Verification items for the finished model (mm, model axes). A direction names the side the tool comes from. Round coordinates to 2 decimals unless told otherwise and drop trailing zeros. Loops run counter-clockwise (first coordinate to the right, second up) from the corner with the lowest first, then second, coordinate; pieces in that order, holes last. Notation, with made-up numbers: (38.25, 28.5) -> (52.25, 28.5) arc R27 ccw to (52.25, 59.5) -> close; hole circle Ø2 at (-10.5, 44). An arc over 180 degrees is marked (long way). Write item = value, one per line. Start each with the question number.
```python
from build123d import *

# Parameters (mm, degrees)
SKETCH1_W           = 63.5
SKETCH1_H           = 38.1
BOSS_EXTRUDE1_DEPTH = 19.05
SHELL1_T            = -2.54
SKETCH2_R           = 1.143
CUT_EXTRUDE1_DEPTH  = 54.127911685
SKETCH4_W           = 7.62
SKETCH4_H           = 12.842115784
CUT_EXTRUDE2_DEPTH  = 54.127911685
SKETCH5_R           = 2.667
CUT_EXTRUDE3_DEPTH  = 54.127911685
SKETCH6_W           = 27.94
SKETCH6_H           = 27.94
CUT_EXTRUDE4_DEPTH  = 69.978656119


with BuildPart() as part:
    # Sketch1 → Boss-Extrude1 (new, symmetric)
    with BuildSketch(Plane.XY):
        Rectangle(SKETCH1_W, SKETCH1_H)
    extrude(amount=BOSS_EXTRUDE1_DEPTH, both=True)

    # Shell1
    shell1_openings = [part.faces().sort_by_distance(p)[0] for p in [
        (0, -19.05, 0),
    ]]
    offset(amount=SHELL1_T, openings=shell1_openings, kind=Kind.INTERSECTION)

    # Sketch2 → Cut-Extrude1 (cut, through all)
    with BuildSketch(Plane(origin=(0, 19.05, 0), x_dir=(1, 0, 0), z_dir=(0, 1, 0))):
        with Locations(Location((-1.27, 10.414, 0), (0, 0, 270))):
            Circle(SKETCH2_R)
        with Locations(Location((21.59, 10.414, 0), (0, 0, 270))):
            Circle(SKETCH2_R)
        with Locations(Location((21.59, -10.414, 0), (0, 0, 270))):
            Circle(SKETCH2_R)
        with Locations(Location((-1.27, -10.414, 0), (0, 0, 270))):
            Circle(SKETCH2_R)
    extrude(amount=-CUT_EXTRUDE1_DEPTH, mode=Mode.SUBTRACT)

    # Sketch4 → Cut-Extrude2 (cut, through all)
    with BuildSketch(Plane(origin=(0, 19.05, 0), x_dir=(1, 0, 0), z_dir=(0, 1, 0))):
        with Locations((-21.59, 0)):
            Rectangle(SKETCH4_W, SKETCH4_H)
    extrude(amount=-CUT_EXTRUDE2_DEPTH, mode=Mode.SUBTRACT)

    # Sketch5 → Cut-Extrude3 (cut, through all)
    with BuildSketch(Plane.XY.offset(19.05)):
        with Locations((-12.7, 0)):
            Circle(SKETCH5_R)
    extrude(amount=-CUT_EXTRUDE3_DEPTH, mode=Mode.SUBTRACT)

    # Sketch6 → Cut-Extrude4 (cut, through all)
    with BuildSketch(Plane.ZY.offset(31.75)):
        Rectangle(SKETCH6_W, SKETCH6_H)
    extrude(amount=-CUT_EXTRUDE4_DEPTH, mode=Mode.SUBTRACT)


solid = part.part
```
(1) Section check B-B on z = 1.5. Enter the section's corners in (x, y), then the cut area to 3 significant figures.
(2) Depth check by flat-ended pin: pin 1 Ø1.4 at (x, z) = (21.59, 10.414) entering from +Y; pin 2 Ø8 at (x, z) = (16.5, 7) entering from -Y. Enter the tip coordinate at first touch or a pass-through.
(3) Access from +Z, -Z, +X, -X, +Y, -Y to the whole of each face (thin tool, end or side, straight path). Record for faces 4 (the flat face through (-17.78, 18, 0)), 5 (the flat face through (30, 0, -13.97)), 6 (the flat face through (0, -1, -16.51)).
(4) Section check C-C on y = 0. Enter the section's corners in (x, z), then the cut area to 3 significant figures.
(5) Section check A-A on x = -12.7. Enter the section's corners in (y, z), then the cut area to 3 significant figures.
(6) Section check D-D on y = 5. Enter the section's corners in (x, z), then the cut area to 3 significant figures.
(7) Scan lines: line 1 (X direction, y = -5, z = -16); line 2 (Z direction, x = -6, y = -7); line 3 (Z direction, x = 21, y = 17). Record each from-to range of solid material in increasing order. Write a range as [from, to].
(8) Draft check along X on faces 1 (the flat face through (-22, 18, -6.421)), 2 (the flat face through (31.75, -17, 0)), 3 (the flat face through (0, 19.05, 0)). Enter one of: +X half, -X half, draft (parallel to the pull), parting line (faces both ways), or undercut.
Computed values:
q1.outline = (-31.75, -19.05) -> (-29.21, -19.05) -> (-29.21, -13.97) -> (-31.75, -13.97) -> close; (-31.75, 13.97) -> (-29.21, 13.97) -> (-29.21, 16.51) -> (-25.4, 16.51) -> (-25.4, 19.05) -> (-31.75, 19.05) -> close; (-17.78, 16.51) -> (29.21, 16.51) -> (29.21, 13.97) -> (31.75, 13.97) -> (31.75, 19.05) -> (-17.78, 19.05) -> close; (29.21, -19.05) -> (31.75, -19.05) -> (31.75, -13.97) -> (29.21, -13.97) -> close
q1.area = 181 mm²
q2.pin_1 = through
q2.pin_2 = 16.51
q3.face_4 = +Y, -Y
q3.face_5 = +X, -X
q3.face_6 = -Y
q4.outline = (-31.75, -19.05) -> (-15.37, -19.05) -> (-15.37, -16.51) -> (-29.21, -16.51) -> (-29.21, -13.97) -> (-31.75, -13.97) -> close; (-31.75, 13.97) -> (-29.21, 13.97) -> (-29.21, 16.51) -> (-15.37, 16.51) -> (-15.37, 19.05) -> (-31.75, 19.05) -> close; (-10.03, -19.05) -> (31.75, -19.05) -> (31.75, -13.97) -> (29.21, -13.97) -> (29.21, -16.51) -> (-10.03, -16.51) -> close; (-10.03, 16.51) -> (29.21, 16.51) -> (29.21, 13.97) -> (31.75, 13.97) -> (31.75, 19.05) -> (-10.03, 19.05) -> close
q4.area = 321 mm²
q5.outline = (-19.05, -19.05) -> (-2.67, -19.05) -> (-2.67, -16.51) -> (-19.05, -16.51) -> close; (-19.05, 16.51) -> (-2.67, 16.51) -> (-2.67, 19.05) -> (-19.05, 19.05) -> close; (2.67, -19.05) -> (19.05, -19.05) -> (19.05, 19.05) -> (2.67, 19.05) -> (2.67, 16.51) -> (16.51, 16.51) -> (16.51, -16.51) -> (2.67, -16.51) -> close
q5.area = 250 mm²
q6.outline = (-31.75, -19.05) -> (31.75, -19.05) -> (31.75, -13.97) -> (29.21, -13.97) -> (29.21, -16.51) -> (-29.21, -16.51) -> (-29.21, -13.97) -> (-31.75, -13.97) -> close; (-31.75, 13.97) -> (-29.21, 13.97) -> (-29.21, 16.51) -> (29.21, 16.51) -> (29.21, 13.97) -> (31.75, 13.97) -> (31.75, 19.05) -> (-31.75, 19.05) -> close
q6.area = 348 mm²
q7.line_1 = [-31.75, -29.21], [29.21, 31.75]
q7.line_2 = [-19.05, -16.51], [16.51, 19.05]
q7.line_3 = [-19.05, -11.39], [-9.44, 9.44], [11.39, 19.05]
q8.face_1 = undercut
q8.face_2 = +X half
q8.face_3 = draft
